```python
from build123d import *

# Parameters (mm, degrees)
EXTRUSION4_DEPTH = 25.4


with BuildPart() as part:
    # Sketch1 → Extrusion4 (new body)
    with BuildSketch(Plane.XY):
        with BuildLine():
            Line((-15.222428705, 14.999999974), (-4.099998637, 14.999999974))
            Line((-4.099998637, 14.999999974), (-4.099998631, 12.499999975))
            Line((-4.099998631, 12.499999975), (-6.799995581, 12.499999968))
            Line((-6.799995581, 12.499999968), (-6.79999557, 7.860655568))
            Line((-6.79999557, 7.860655568), (-3.941498133, 5.002158145))
            Line((-3.941498133, 5.002158145), (3.941497857, 5.002158165))
            Line((3.941497857, 5.002158165), (6.79999528, 7.860655602))
            Line((6.79999528, 7.860655602), (6.799995269, 12.500000002))
            Line((6.799995269, 12.500000002), (4.099998319, 12.499999995))
            Line((4.099998319, 12.499999995), (4.099998313, 14.999999995))
            Line((4.099998313, 14.999999995), (14.92634643, 15.000000022))
            ThreePointArc((14.92634643, 15.000000022), (14.981582716, 13.713730334), (14.999999839, 12.426406922))
            ThreePointArc((14.999999839, 12.426406922), (11.574578842, -4.794347555), (1.819805062, -19.393398286))
            ThreePointArc((1.819805062, -19.393398286), (0.896507077, -20.290650536), (-0.052080894, -21.161122609))
            Line((-0.052080894, -21.161122609), (-7.707465087, -13.505738454))
            Line((-7.707465087, -13.505738454), (-5.939698141, -11.7379715))
            Line((-5.939698141, -11.7379715), (-4.030511986, -13.647157645))
            Line((-4.030511986, -13.647157645), (-0.750000115, -10.366645757))
            Line((-0.750000115, -10.366645757), (-0.750000125, -6.324119927))
            Line((-0.750000125, -6.324119927), (-6.324120058, -0.75000002))
            Line((-6.324120058, -0.75000002), (-10.366645888, -0.75000003))
            Line((-10.366645888, -0.75000003), (-13.64715776, -4.030511919))
            Line((-13.64715776, -4.030511919), (-11.737971606, -5.939698064))
            Line((-11.737971606, -5.939698064), (-13.505738551, -7.707465018))
            Line((-13.505738551, -7.707465018), (-21.370484292, 0.157280684))
            ThreePointArc((-21.370484292, 0.157280684), (-20.34608634, 0.945903864), (-19.393398415, 1.819805117))
            ThreePointArc((-19.393398415, 1.819805117), (-16.141807163, 6.68615536), (-15.000000161, 12.426406848))
            ThreePointArc((-15.000000161, 12.426406848), (-15.055710753, 13.718000441), (-15.222428705, 14.999999974))
        make_face()
        with BuildLine():
            Line((-4.031774412, 0.587623385), (-4.381628794, 1.432246584))
            ThreePointArc((-4.381628794, 1.432246584), (-4.381628794, 1.814930015), (-4.111030745, 2.085528065))
            Line((-4.111030745, 2.085528065), (-3.266407566, 2.435382447))
            Line((-3.266407566, 2.435382447), (-3.161030076, 2.391733657))
            ThreePointArc((-3.161030076, 2.391733657), (-2.978032474, 2.376750688), (-2.820578756, 2.471201408))
            ThreePointArc((-2.820578756, 2.471201408), (-0.731588872, 3.677944803), (1.660186832, 3.362481109))
            ThreePointArc((1.660186832, 3.362481109), (1.841799821, 3.33547495), (2.005133821, 3.41934756))
            Line((2.005133821, 3.41934756), (2.085786261, 3.5))
            Line((2.085786261, 3.5), (2.999999821, 3.500000003))
            ThreePointArc((2.999999821, 3.500000003), (3.353553212, 3.353553393), (3.499999822, 3.000000004))
            Line((3.499999822, 3.000000004), (3.499999825, 2.085786444))
            Line((3.499999825, 2.085786444), (3.419347385, 2.005134004))
            ThreePointArc((3.419347385, 2.005134004), (3.335474775, 1.841800003), (3.362480936, 1.660187013))
            ThreePointArc((3.362480936, 1.660187013), (3.464548079, -1.435062852), (1.203703559, -3.551562652))
            ThreePointArc((1.203703559, -3.551562652), (1.056187548, -3.660886193), (0.999999859, -3.835687662))
            Line((0.999999859, -3.835687662), (0.99999986, -3.949747432))
            Line((0.99999986, -3.949747432), (0.353553251, -4.596194044))
            ThreePointArc((0.353553251, -4.596194044), (-1.38e-07, -4.742640655), (-0.353553529, -4.596194046))
            Line((-0.353553529, -4.596194046), (-1.00000014, -3.949747437))
            Line((-1.00000014, -3.949747437), (-1.000000141, -3.835687667))
            ThreePointArc((-1.000000141, -3.835687667), (-1.056187824, -3.660886194), (-1.203703841, -3.551562658))
            ThreePointArc((-1.203703841, -3.551562658), (-3.118011196, -2.083388382), (-3.741853671, 0.247046976))
            ThreePointArc((-3.741853671, 0.247046976), (-3.786403511, 0.425170315), (-3.926396922, 0.543974595))
            Line((-3.926396922, 0.543974595), (-4.031774412, 0.587623385))
        make_face(mode=Mode.SUBTRACT)
        with BuildLine():
            Line((7.799995261, 7.567762394), (7.799995245, 14.000000024))
            Line((7.799995245, 14.000000024), (13.971852229, 14.00000004))
            ThreePointArc((13.971852229, 14.00000004), (13.992962358, 13.213329344), (13.999999819, 12.426406924))
            ThreePointArc((13.999999819, 12.426406924), (13.273442442, 4.463419684), (11.117765058, -3.236587227))
            ThreePointArc((11.117765058, -3.236587227), (10.848477439, -3.517741288), (10.459176009, -3.520538429))
            Line((10.459176009, -3.520538429), (5.472273453, -1.454895771))
            ThreePointArc((5.472273453, -1.454895771), (5.225369073, -1.233664041), (5.171126882, -0.906612002))
            ThreePointArc((5.171126882, -0.906612002), (5.246544564, 0.190443263), (5.091786587, 1.279143428))
            ThreePointArc((5.091786587, 1.279143428), (5.115772732, 3.31925596), (6.142816007, 5.08215601))
            Line((6.142816007, 5.08215601), (7.214208825, 6.153548833))
            ThreePointArc((7.214208825, 6.153548833), (7.647754322, 6.802395532), (7.799995261, 7.567762394))
        make_face(mode=Mode.SUBTRACT)
        with BuildLine():
            Line((0.749999883, -9.452432163), (0.749999879, -7.937253913))
            ThreePointArc((0.749999879, -7.937253913), (1.270329188, -5.964466066), (2.695945821, -4.504927888))
            ThreePointArc((2.695945821, -4.504927888), (3.575203493, -3.84453103), (4.297610347, -3.01546746))
            ThreePointArc((4.297610347, -3.01546746), (4.567226078, -2.822561759), (4.898248297, -2.840715069))
            Line((4.898248297, -2.840715069), (9.885150852, -4.906357727))
            ThreePointArc((9.885150852, -4.906357727), (10.158450647, -5.183613277), (10.150059814, -5.57283431))
            ThreePointArc((10.150059814, -5.57283431), (6.229626845, -12.541855522), (1.112698256, -18.686291472))
            ThreePointArc((1.112698256, -18.686291472), (0.551283843, -19.237753416), (-0.019903451, -19.779086485))
            Line((-0.019903451, -19.779086485), (-4.384065382, -15.414924576))
            Line((-4.384065382, -15.414924576), (0.164213447, -10.866645724))
            ThreePointArc((0.164213447, -10.866645724), (0.597758953, -10.217799029), (0.749999883, -9.452432163))
        make_face(mode=Mode.SUBTRACT)
        with BuildLine():
            Line((-14.07756929, 13.99999997), (-7.799995595, 13.999999986))
            Line((-7.799995595, 13.999999986), (-7.799995579, 7.567762366))
            ThreePointArc((-7.799995579, 7.567762366), (-7.647754645, 6.802395501), (-7.214209135, 6.153548807))
            Line((-7.214209135, 6.153548807), (-6.078427273, 5.01776695))
            ThreePointArc((-6.078427273, 5.01776695), (-5.536495387, 2.29329142), (-7.846194212, 0.749999996))
            Line((-7.846194212, 0.749999996), (-9.452432322, 0.749999992))
            ThreePointArc((-9.452432322, 0.749999992), (-10.217799187, 0.597759058), (-10.866645881, 0.164213548))
            Line((-10.866645881, 0.164213548), (-15.414924709, -4.384065303))
            Line((-15.414924709, -4.384065303), (-19.853839651, 0.054849617))
            ThreePointArc((-19.853839651, 0.054849617), (-19.257037077, 0.569394344), (-18.686291624, 1.112698328))
            ThreePointArc((-18.686291624, 1.112698328), (-15.217927205, 6.303472924), (-14.000000151, 12.426409013))
            ThreePointArc((-14.000000151, 12.426409013), (-14.019404256, 13.214159839), (-14.07756929, 13.99999997))
        make_face(mode=Mode.SUBTRACT)
    extrude(amount=EXTRUSION4_DEPTH)


solid = part.part
```
Design review of the part built by this model. Coordinates are the model's own, in mm. A direction names the side the tool comes from. Coordinates: 2 decimals unless noted, no trailing zeros. Loops run counter-clockwise (first coordinate to the right, second up) from the corner with the lowest first, then second, coordinate; pieces in that order, holes last.
Q1. For pin 1 (3 mm diameter, centred on y = 12, z = 18, fed in from -X); pin 2 (6 mm diameter, centred on y = 8.5, z = 19, fed in from -X); pin 3 (1.4 mm diameter, centred on y = 9, z = 18.5, fed in from -X); pin 4 (3 mm diameter, centred on x = -8, y = -3, fed in from +Z), all flat-tipped, find the tip position at first contact; note any pin that passes through.
Reported:
pin 1: stops at x = -15.12
pin 2: stops at x = -16.69
pin 3: stops at x = -15.58
pin 4: passes through
Q2. We need section B-B on x = -13. State the section outline as (y, z) points, and give its area (3 significant figures).
Reported:
outline: (-7.2, 0) - (-4.68, 0) - (-4.68, 25.4) - (-7.2, 25.4) - close; (-3.38, 0) - (-1.97, 0) - (-1.97, 25.4) - (-3.38, 25.4) - close; (14, 0) - (15, 0) - (15, 25.4) - (14, 25.4) - close
area: 125 mm2
Q3. We need section D-D on z = 16. State how many separate pieces and enclosed holes the cut face has, and give its area (3 significant figures).
Reported:
separate pieces: 1
enclosed holes: 4
area: 226 mm2
Q4. We need section C-C on x = 12.5. State the section outline as (y, z) points, and give its area (3 significant figures).
Reported:
outline: (-2.36, 0) - (1.04, 0) - (1.04, 25.4) - (-2.36, 25.4) - close; (14, 0) - (15, 0) - (15, 25.4) - (14, 25.4) - close
area: 112 mm2
Q5. Tool access review of faces 3 (the face through (-5, 12.5, 13)), 4 (the face through (-2, 4, 25.4)): name each direction out of +Z, -Z, +X, -X, +Y, -Y from which nothing blocks a thin tool from reaching the whole face with its end or side.
Reported:
face 3: +Z, -Z
face 4: +Z, +X, -X, +Y, -Y
Q6. We need section A-A on y = -16. State the section outline as (x, z) points, and give its area (3 significant figures).
Reported:
outline: (-5.21, 0) - (-3.8, 0) - (-3.8, 25.4) - (-5.21, 25.4) - close; (3.58, 0) - (4.88, 0) - (4.88, 25.4) - (3.58, 25.4) - close
area: 68.9 mm2
Q7. To check wall thickness, follow line 1 (Y direction, x = 9, z = 19.5); line 2 (X direction, y = -6, z = 12.75); line 3 (X direction, y = 7, z = 8). State the ranges of each line that lie inside material, in increasing order.
Reported:
line 1: y = -10.02 to -7.95, -4.54 to -2.92, 14 to 15
line 2: x = -15.21 to -11.8, -1.07 to 1.25, 9.96 to 11.05
line 3: x = -16.02 to -14.95, -7.72 to -5.94, 5.94 to 7.72, 13.66 to 14.67
Q8. The part is to be moulded in two halves that separate along X. For faces 1 (the face through (9, 15, 13)), 2 (the face through (2.5, 3.5, 12.5)), say which applies: +X half, -X half, draft (parallel to the pull), parting line (faces both ways), or undercut.
Reported:
face 1: draft
face 2: undercut
